Could you check a few things on this model? Use its own coordinates, in mm. Face numbers are marked on the shaded views. A direction names the side the tool comes from. Give positions to 0.01 mm unless a question says otherwise; leave off trailing zeros. Order: outer loops, then holes, each group sorted by start corner. A loop starts at its lowest first (then second) coordinate and runs counter-clockwise, first axis right, second up. Notation, with made-up numbers: (64, 31.5) -> (84, 31.5) arc R23 cw to (84, 54.5) -> close; hole circle Ø9 at (-32, 78). An arc over 180 degrees is marked (long way). One line per item, written item: value.
```python
from build123d import *

# Parameters (mm, degrees)
SKETCH1_W           = 40
SKETCH1_H           = 40
SKETCH1_W_2         = 36
SKETCH1_H_2         = 36
EXTRUDE_THIN1_DEPTH = 380
SKETCH2_R           = 2.5
CUT_EXTRUDE1_DEPTH  = 50
SKETCH3_R           = 2.5
CUT_EXTRUDE2_DEPTH  = 50


with BuildPart() as part:
    # Sketch1 → Extrude-Thin1 (new body)
    with BuildSketch(Plane(origin=(0, 0, 0), x_dir=(1, 0, 0), z_dir=(0, 1, 0))):
        with Locations((-20, 20)):
            Rectangle(SKETCH1_W, SKETCH1_H)
        with Locations((-20, 20)):
            Rectangle(SKETCH1_W_2, SKETCH1_H_2, mode=Mode.SUBTRACT)
    extrude(amount=EXTRUDE_THIN1_DEPTH)

    # Sketch2 → Cut-Extrude1 (cut)
    with BuildSketch(Plane.XY):
        with Locations((-20, 357.5)):
            Circle(SKETCH2_R)
    extrude(amount=-CUT_EXTRUDE1_DEPTH, mode=Mode.SUBTRACT)

    # Sketch3 → Cut-Extrude2 (cut)
    with BuildSketch(Plane.ZY.offset(40)):
        with Locations((-20, 14)):
            Circle(SKETCH3_R)
        with Locations((-20, 74)):
            Circle(SKETCH3_R)
    extrude(amount=-CUT_EXTRUDE2_DEPTH, mode=Mode.SUBTRACT)


solid = part.part
```
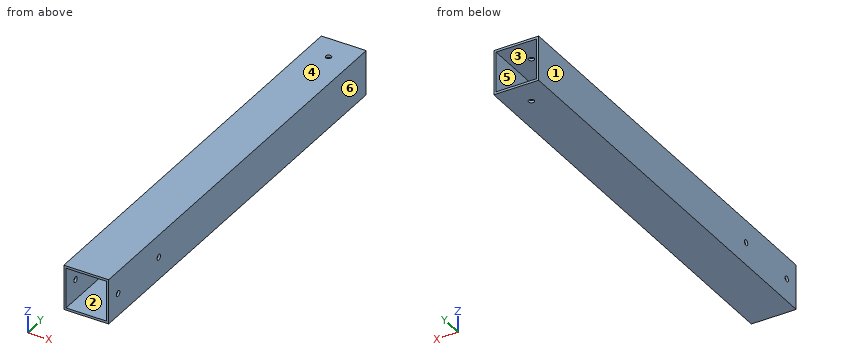
1) Suppose I cut it at A-A, the plane y = 155. Write out the boundary of the cut face in (x, z).
Answer below:
outline: (-40, -40) -> (0, -40) -> (0, 0) -> (-40, 0) -> close; hole (-38, -38) -> (-2, -38) -> (-2, -2) -> (-38, -2) -> close
2) For the marked faces 5 and 6, which set-ups out of +Z, -Z, +X, -X, +Y, -Y let a thin tool reach every point of the face, with its end or its side?
Answer below:
face 5: +Y, -Y
face 6: +Z, -Z, +X, +Y, -Y
3) For P1, Ø6, axis at y = 260, z = -24, coming from the +X side, with a flat end and sliding along its axis, tell me the tip position at first contact or that it passes through.
Answer below:
P1: stops at x = 0
4) We'd pull the mould along X, two halves only. Please class the marked faces 1, 2, 3 and 4: +X half, -X half, draft (parallel to the pull), parting line (faces both ways), or undercut.
Answer below:
face 1: -X half
face 2: undercut
face 3: undercut
face 4: draft
5) Suppose I cut it at B-B, the plane x = -30. Write out the boundary of the cut face in (y, z), then the cut area to 3 significant figures.
Answer below:
outline: (0, -40) -> (380, -40) -> (380, -38) -> (0, -38) -> close; (0, -2) -> (380, -2) -> (380, 0) -> (0, 0) -> close
area: 1,520 mm2
6) If I drill on line 1 along Y through (x, z) = (-1, -20); line 2 along X through (y, z) = (340, -20), over which ranges is the centre line in solid material (lowest first)?
Answer below:
line 1: y = 0 to 11.5, 16.5 to 71.5, 76.5 to 380
line 2: x = -40 to -38, -2 to 0
